Answer from the drawing. Dimensions are ordinates in mm from the lowest x, y and z of the part. A direction names the side the tool comes from. Coordinates: 2 decimals unless noted, no trailing zeros. Loops run counter-clockwise (first coordinate to the right, second up) from the corner with the lowest first, then second, coordinate; pieces in that order, holes last. Notation, with made-up numbers: (8.25, 14) - (26.25, 14) arc R18 cw to (26.25, 43) - close; hole circle Ø11 at (-11, -29.5). An arc over 180 degrees is marked (long way). Write each question's results on one line, items separated by ' | '. Start each with the question number.
1. A cutting plane is placed at D-D on x = 19.5. Determine the outline of the cut face in (y, z), then the cut area to 3 significant figures.
2. Each of these flat-tipped pins is pushed along its axis until it touches: P1, Ø1.2, axis at y = 2.5, z = 6, coming from the +X side; P2, Ø12, axis at y = 17.5, z = 16.5, coming from the +X side. Where does it stop, or does it pass through?
3. A cutting plane is placed at B-B on x = 2.45. Determine the outline of the cut face in (y, z), then the cut area to 3 significant figures.
4. Which of the six approach directions +Z, -Z, +X, -X, +Y, -Y give full straight-line access (tool end or side, diameter ignored) to the marked faces 1, 2 and 3?
5. Find the intervals of material crossed by line 1 along Z through (x, y) = (2.45, 19.9); line 2 along X through (y, z) = (16.25, 12), in increasing order. Write a range as [from, to].
6. Determine the mould class of the marked faces 4, 5 and 6 for opening direction Z: released by +Z, released by -Z, zero draft, split by the parting line, or undercut.
7. A cutting plane is placed at A-A on z = 15.75. Determine the outline of the cut face in (x, y), then the cut area to 3 significant figures.
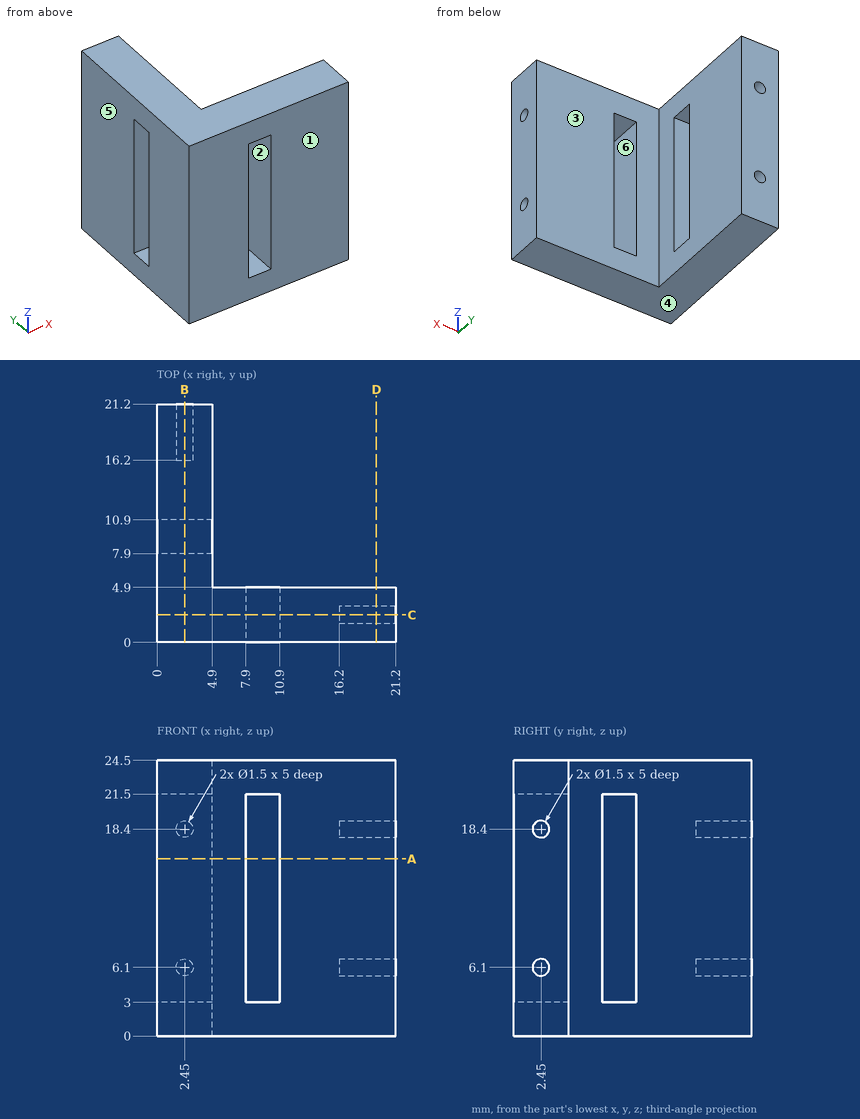
Values:
1) outline: (0, 0) - (4.9, 0) - (4.9, 24.5) - (0, 24.5) - close; hole circle Ø1.5 at (2.45, 6.1); hole circle Ø1.5 at (2.45, 18.4) | area: 117 mm^2
2) P1: x = 16.2 | P2: x = 4.9
3) outline: (0, 0) - (21.2, 0) - (21.2, 5.35) - (16.2, 5.35) - (16.2, 6.85) - (21.2, 6.85) - (21.2, 17.65) - (16.2, 17.65) - (16.2, 19.15) - (21.2, 19.15) - (21.2, 24.5) - (0, 24.5) - close; hole (7.9, 3) - (10.9, 3) - (10.9, 21.5) - (7.9, 21.5) - close | area: 449 mm^2
4) face 1: +Z, -Z, +X, -X, -Y | face 2: +Y, -Y | face 3: +Z, -Z, +X, +Y
5) line 1: [0, 5.35], [6.85, 17.65], [19.15, 24.5] | line 2: [0, 4.9]
6) face 4: released by -Z | face 5: zero draft | face 6: undercut
7) outline: (0, 0) - (7.9, 0) - (7.9, 4.9) - (4.9, 4.9) - (4.9, 7.9) - (0, 7.9) - close; (0, 10.9) - (4.9, 10.9) - (4.9, 21.2) - (0, 21.2) - close; (10.9, 0) - (21.2, 0) - (21.2, 4.9) - (10.9, 4.9) - close | area: 154 mm^2
